from build123d import *

# Parameters (mm, degrees)
SKETCH1_W           = 25
SKETCH1_H           = 15
BOSS_EXTRUDE1_DEPTH = 3
CUT_EXTRUDE1_DEPTH  = 3
SKETCH3_W           = 3
SKETCH3_H           = 15
BOSS_EXTRUDE2_DEPTH = 12
SKETCH4_R           = 2
CUT_EXTRUDE2_DEPTH  = 12


with BuildPart() as part:
    # Sketch1 → Boss-Extrude1 (new body)
    with BuildSketch(Plane.XY):
        Rectangle(SKETCH1_W, SKETCH1_H)
    extrude(amount=BOSS_EXTRUDE1_DEPTH)

    # Sketch2 → Cut-Extrude1 (cut)
    with BuildSketch(Plane.XY.offset(3)):
        with BuildLine():
            Line((8.5, -2), (-1.947413085, -2))
            ThreePointArc((-1.947413085, -2), (-3.947413085, 0), (-1.947413085, 2))
            Line((-1.947413085, 2), (8.5, 2))
            ThreePointArc((8.5, 2), (10.5, 0), (8.5, -2))
        make_face()
    extrude(amount=-CUT_EXTRUDE1_DEPTH, mode=Mode.SUBTRACT)

    # Sketch3 → Boss-Extrude2 (add)
    with BuildSketch(Plane.XY.offset(3)):
        with Locations((-11, 0)):
            Rectangle(SKETCH3_W, SKETCH3_H)
    extrude(amount=BOSS_EXTRUDE2_DEPTH)

    # Sketch4 → Cut-Extrude2 (cut)
    with BuildSketch(Plane.ZY.offset(12.5)):
        with Locations(Location((7.5, 0, 0), (0, 0, 270))):
            Circle(SKETCH4_R)
    extrude(amount=-CUT_EXTRUDE2_DEPTH, mode=Mode.SUBTRACT)


solid = part.part
Input: part model. Units: mm. Frame: model coordinates. A direction names the side the tool comes from. Coordinates: 2 decimals unless noted, no trailing zeros. Loops run counter-clockwise (first coordinate to the right, second up) from the corner with the lowest first, then second, coordinate; pieces in that order, holes last.
Q1. Cut plane C-C (x = 5.75). Output: boundary loops of the cut face in (y, z), then the cut area to 3 significant figures.
Q2. Set-up query: faces 1 (the face through (-3.947, -0.044, 1.521)), 2 (the face through (-3, 7.5, 2)), 3 (the face through (-9.5, 0, 10)). Return all of +Z, -Z, +X, -X, +Y, -Y with unobstructed straight access to the full face (end or side cutting, diameter ignored); none if empty.
Q3. Material intervals for line 1 (Y direction, x = 3, z = 1.25); line 2 (Z direction, x = -11.05, y = 0); line 3 (X direction, y = -4.5, z = 10), sorted ascending.
Q4. Contact query for flat-ended pins moving along their axis: pin 1 (7.5 mm diameter, centred on x = 1.5, y = 3, fed in from +Z); pin 2 (3.5 mm diameter, centred on y = -1.5, z = 9.5, fed in from +X). Output: stop coordinate, or through.
Q5. Draft query along Z for faces 4 (the face through (-11, 0, 15)), 5 (the face through (-11.021, 0.26, 9.483)), 6 (the face through (-3, 2, 0)), 7 (the face through (3, 2, 2)). Return one class per face: +Z half, -Z half, draft (parallel to the pull), parting line (faces both ways), or undercut.
Q6. Cut plane B-B (y = 0). Output: boundary loops of the cut face in (x, z).
Q7. Cut plane D-D (z = 1.75). Output: boundary loops of the cut face in (x, y), then the cut area to 3 significant figures.
Q8. Cut plane A-A (z = 7.5). Output: boundary loops of the cut face in (x, y).
Working result:
1. outline: (-7.5, 0) - (-2, 0) - (-2, 3) - (-7.5, 3) - close; (2, 0) - (7.5, 0) - (7.5, 3) - (2, 3) - close
1. area: 33.0 mm2
2. face 1: +Z, -Z
2. face 2: +Z, -Z, +X, -X, +Y
2. face 3: +Z, +X, +Y, -Y
3. line 1: y = -7.5 to -2, 2 to 7.5
3. line 2: z = 0 to 5.5, 9.5 to 15
3. line 3: x = -12.5 to -9.5
4. pin 1: stops at z = 3
4. pin 2: stops at x = -9.5
5. face 4: +Z half
5. face 5: undercut
5. face 6: -Z half
5. face 7: draft
6. outline: (-12.5, 0) - (-3.95, 0) - (-3.95, 3) - (-9.5, 3) - (-9.5, 5.5) - (-12.5, 5.5) - close; (-12.5, 9.5) - (-9.5, 9.5) - (-9.5, 15) - (-12.5, 15) - close; (10.5, 0) - (12.5, 0) - (12.5, 3) - (10.5, 3) - close
7. outline: (-12.5, -7.5) - (12.5, -7.5) - (12.5, 7.5) - (-12.5, 7.5) - close; hole (-1.95, -2) - (8.5, -2) arc R2 ccw to (8.5, 2) - (-1.95, 2) arc R2 ccw to start
7. area: 321 mm2
8. outline: (-12.5, -7.5) - (-9.5, -7.5) - (-9.5, -2) - (-12.5, -2) - close; (-12.5, 2) - (-9.5, 2) - (-9.5, 7.5) - (-12.5, 7.5) - close
